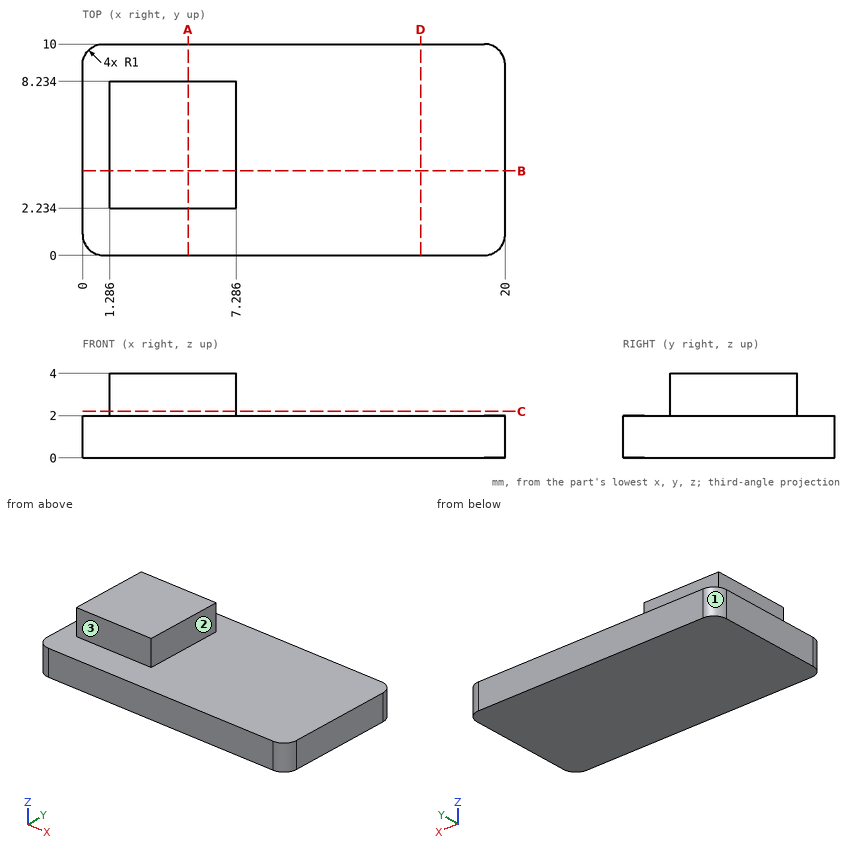
Drawing for the job (mm, zero at the part's lowest x, y, z). A direction names the side the tool comes from. Round coordinates to 2 decimals unless told otherwise and drop trailing zeros. Write each loop counter-clockwise with the first axis right and the second up, starting at its lowest first coordinate (ties: lowest second). Pieces come first, ordered by that corner, then holes. Notation, with made-up numbers: (-13.75, 88) - (23.25, 88) arc R18 ccw to (23.25, 110) - close; hole circle Ø10 at (-35.5, 44). An arc over 180 degrees is marked (long way). Write item = value, one per line. Start each with the question number.
Q1. Band-saw the part on C-C (z = 2.2). Give the cut face in (x, y) (1 decimal), then the cut area to 3 significant figures.
Q2. Band-saw the part on D-D (x = 16). Give the cut face in (y, z), then the cut area to 3 significant figures.
Q3. Which spindle directions (+Z, -Z, +X, -X, +Y, -Y) get a long thin tool onto all of the face, cutting with end or side? Do the marked faces 1, 2 and 3. Say none if no direction does.
Q4. Band-saw the part on B-B (y = 4). Give the cut face in (x, z) (1 decimal).
Q5. Drop flat-ended pins along their axis: pin 1 (0.6 mm diameter, centred on y = 5.5, z = 3.5, fed in from -X) (1 decimal); pin 2 (1.6 mm diameter, centred on x = 3.5, z = 3, fed in from +Y); pin 3 (2 mm diameter, centred on y = 5.5, z = 3.5, fed in from +X) (1 decimal). Give the stop position or say it passes through.
Q6. Band-saw the part on A-A (x = 5). Give the cut face in (y, z).
Q7. Probe L1, parallel to Z at x = 12, y = 3.25; L2, parallel to X at y = 5, z = 2.25 (1 decimal); L3, parallel to Y at x = 6.25, z = 2.2. List the from-to ranges inside material, lowest first. Write a range as from..to.
Answers below:
q1.outline = (1.3, 2.2) - (7.3, 2.2) - (7.3, 8.2) - (1.3, 8.2) - close
q1.area = 36.0 mm2
q2.outline = (0, 0) - (10, 0) - (10, 2) - (0, 2) - close
q2.area = 20.0 mm2
q3.face_1 = +Z, -Z, -X, +Y
q3.face_2 = +Z, +X, +Y, -Y
q3.face_3 = +Z, +X, -X, -Y
q4.outline = (0, 0) - (20, 0) - (20, 2) - (7.3, 2) - (7.3, 4) - (1.3, 4) - (1.3, 2) - (0, 2) - close
q5.pin_1 = 1.3
q5.pin_2 = 8.23
q5.pin_3 = 7.3
q6.outline = (0, 0) - (10, 0) - (10, 2) - (8.23, 2) - (8.23, 4) - (2.23, 4) - (2.23, 2) - (0, 2) - close
q7.L1 = 0..2
q7.L2 = 1.3..7.3
q7.L3 = 2.23..8.23
